from build123d import *

# Parameters (mm, degrees)
F0_W     = 105.0036
F0_H     = 24.9936
F1_DEPTH = 21.9964
F3_DEPTH = 1.5875
F4_R     = 1.5875
F5_R     = 3.175
F6_W     = 105.034594
F6_H     = 24.9936
F6_W_2   = 96.52
F6_H_2   = 15.748
F7_DEPTH = 0.508


with BuildPart() as f1:
    # F0 (on Top) → F1 (new body)
    with BuildSketch(Plane.XY):
        with Locations((-52.5018, 12.4968)):
            Rectangle(F0_W, F0_H)
    extrude(amount=F1_DEPTH)

    # F2 (on face) → F3 (join)
    with BuildSketch(Plane.XY.offset(21.9964)):
        with BuildLine():
            Line((-111.3536, 18.8468), (-158.9786, 18.8468))
            ThreePointArc((-158.9786, 18.8468), (-165.3286, 12.4968), (-158.9786, 6.1468))
            Line((-158.9786, 6.1468), (-111.3536, 6.1468))
            Line((-111.3536, 6.1468), (-106.5911, 0))
            Line((-106.5911, 0), (-105.0036, 0))
            Line((-105.0036, 0), (-105.0036, 1.5875))
            Line((-105.0036, 1.5875), (-105.812847, 1.5875))
            Line((-105.812847, 1.5875), (-110.575347, 7.7343))
            Line((-110.575347, 7.7343), (-158.978601, 7.7343))
            ThreePointArc((-158.978601, 7.7343), (-163.7411, 12.4968), (-158.9786, 17.2593))
            Line((-158.9786, 17.2593), (-110.575347, 17.2593))
            Line((-110.575347, 17.2593), (-105.812847, 23.4061))
            Line((-105.812847, 23.4061), (-105.0036, 23.4061))
            Line((-105.0036, 23.4061), (-105.0036, 24.9936))
            Line((-105.0036, 24.9936), (-106.5911, 24.9936))
            Line((-106.5911, 24.9936), (-111.3536, 18.8468))
        make_face()
    extrude(amount=-F3_DEPTH)

    # F4
    f4_edges = [f1.edges().sort_by_distance(p)[0] for p in [
        (-111.3536, 18.8468, 21.20265),
        (-105.812847, 23.4061, 21.20265),
        (-111.3536, 6.1468, 21.20265),
        (-105.812847, 1.5875, 21.20265),
    ]]
    fillet(f4_edges, radius=F4_R)

    # F5
    f5_edges = [f1.edges().sort_by_distance(p)[0] for p in [
        (-110.575347, 7.7343, 21.20265),
        (-106.5911, 24.9936, 21.20265),
        (-110.575347, 17.2593, 21.20265),
        (-106.5911, 0, 21.20265),
    ]]
    fillet(f5_edges, radius=F5_R)

    # F6 (on face) → F7 (join)
    with BuildSketch(Plane.XY.offset(21.9964)):
        with Locations((-52.517297, 12.4968)):
            Rectangle(F6_W, F6_H)
        with Locations((-52.517554, 12.4968)):
            Rectangle(F6_W_2, F6_H_2, mode=Mode.SUBTRACT)
    extrude(amount=F7_DEPTH)


solid = f1.part
Build history of the part. All positions in model axes, mm. A direction names the side the tool comes from. Round coordinates to 2 decimals unless told otherwise and drop trailing zeros. Order: outer loops, then holes, each group sorted by start corner. A loop starts at its lowest first (then second) coordinate and runs counter-clockwise, first axis right, second up. Notation, with made-up numbers: M 33.25,-37.75 L 60.25,-37.75 A28 cw 60.25,0.25 Z; hole C 34,13 d7. An arc over 180 degrees is marked long. Use CSV: the item, a comma, the result in double quotes. Start each with the question number.
(1) Tool access for faces 4 (the face through (-135, 18, 20.409)), 5 (the face through (-53, 13, 21.996)), 6 (the face through (-135, 18, 21.996)), 7 (the face through (-163.74, 12.39, 21.21)): list every direction of +Z, -Z, +X, -X, +Y, -Y with a clear straight run to the whole face (end or side of a thin tool).
(2) Cut at C-C on z = 2.25. List the corners of the cut face in (x, y).
(3) Mould opens along X. For faces 1 (the face through (-109.234, 3.411, 21.214)), 2 (the face through (-107.98, 20.61, 21.21)), 3 (the face through (-53, 4, 22.504)) say: +X half, -X half, draft (parallel to the pull), parting line (faces both ways), or undercut.
(4) Cut at A-A on x = -151. List the corners of the cut face in (y, z), then the cut area to 3 significant figures.
(5) Drill centre lines: probe 1 along X at (y, z) = (16.25, 14.5); probe 2 along Z at (x, y) = (-77.5, 13.75); probe 3 along Z at (x, y) = (-123.5, 18.75). Where is each one in solid material? Low to high.
(6) Flat gauge pins, fed straight in: P1, Ø1.3, axis at x = -124.5, z = 21.5, coming from the +Y side; P2, Ø0.8, axis at x = -147.5, z = 21, coming from the -Y side; P3, Ø11, axis at y = 17, z = 11, coming from the -X side; P4, Ø10, axis at x = -83, z = 18.5, coming from the -Y side. Where does each tip first touch, or does it go through?
Findings:
1,face 4,"-Z, -X, +Y, -Y"
1,face 5,"+Z"
1,face 6,"+Z, -X, +Y, -Y"
1,face 7,"+Z, -Z"
2,outline,"M -105,0 L 0,0 L 0,24.99 L -105,24.99 Z"
3,face 1,"-X half"
3,face 2,"undercut"
3,face 3,"draft"
4,outline,"M 6.15,20.41 L 7.73,20.41 L 7.73,22 L 6.15,22 Z; M 17.26,20.41 L 18.85,20.41 L 18.85,22 L 17.26,22 Z"
4,area,"5.04 mm^2"
5,probe 1,"x = -105 to 0"
5,probe 2,"z = 0 to 22"
5,probe 3,"z = 20.41 to 22"
6,P1,"stops at y = 18.85"
6,P2,"stops at y = 6.15"
6,P3,"stops at x = -105"
6,P4,"stops at y = 0"
